For this review, take the finished solid that the model builds, in its own axes (mm). Give positions to 0.01 mm unless a question says otherwise; leave off trailing zeros. Write each loop counter-clockwise with the first axis right and the second up, starting at its lowest first coordinate (ties: lowest second). Pieces come first, ordered by that corner, then holes. Notation, with made-up numbers: (82, 72.25) -> (139, 72.25) arc R24 cw to (139, 105.25) -> close; hole circle Ø7 at (78, 54). An arc over 180 degrees is marked (long way). Answer as CSV lines item,"result".
```python
from build123d import *

# Parameters (mm, degrees)
SKETCH1_W                                          = 176.276
SKETCH1_H                                          = 49.149
BOSS_EXTRUDE1_DEPTH                                = 6.35
CUT_EXTRUDE3_DEPTH                                 = 92.719875677
CSK_FOR_10_FLAT_HEAD_MACHINE_SCREW_100_D           = 5.1054
CSK_FOR_10_FLAT_HEAD_MACHINE_SCREW_100_CSINK_D     = 9.779
CSK_FOR_10_FLAT_HEAD_MACHINE_SCREW_100_CSINK_ANGLE = 100


with BuildPart() as part:
    # Sketch1 → Boss-Extrude1 (new body)
    with BuildSketch(Plane.XY):
        Rectangle(SKETCH1_W, SKETCH1_H)
    extrude(amount=BOSS_EXTRUDE1_DEPTH)

    # Sketch22 → Cut-Extrude3 (cut, through all)
    with BuildSketch(Plane.XY.offset(6.35)):
        with BuildLine():
            ThreePointArc((-88.138, 2.504831531), (-81.209963357, 17.310760321), (-66.565807357, 24.5745))
            Line((-66.565807357, 24.5745), (-88.138, 24.5745))
            Line((-88.138, 24.5745), (-88.138, 2.504831531))
        make_face()
        with BuildLine():
            ThreePointArc((-66.565807357, -24.5745), (-81.209963357, -17.310760321), (-88.138, -2.504831531))
            Line((-88.138, -2.504831531), (-88.138, -24.5745))
            Line((-88.138, -24.5745), (-66.565807357, -24.5745))
        make_face()
        with BuildLine():
            Line((88.138, -24.5745), (88.138, -2.504831531))
            ThreePointArc((88.138, -2.504831531), (81.209963357, -17.310760321), (66.565807357, -24.5745))
            Line((66.565807357, -24.5745), (88.138, -24.5745))
        make_face()
        with BuildLine():
            Line((88.138, 24.5745), (66.565807357, 24.5745))
            ThreePointArc((66.565807357, 24.5745), (81.209963357, 17.310760321), (88.138, 2.504831531))
            Line((88.138, 2.504831531), (88.138, 24.5745))
        make_face()
    extrude(amount=-CUT_EXTRUDE3_DEPTH, mode=Mode.SUBTRACT)

    # CSK for #10 Flat Head Machine Screw (100)1 (through all)
    with Locations(Plane.XY.offset(6.35)):
        with Locations((-66.565807357, 19.4945), (-33.282903678, 19.4945), (0, 19.4945), (33.282903678, 19.4945), (66.565807357, 19.4945), (66.565807357, -19.4945), (33.282903678, -19.4945), (0, -19.4945), (-33.282903678, -19.4945), (-66.565807357, -19.4945)):
            CounterSinkHole(CSK_FOR_10_FLAT_HEAD_MACHINE_SCREW_100_D / 2, CSK_FOR_10_FLAT_HEAD_MACHINE_SCREW_100_CSINK_D / 2, counter_sink_angle=CSK_FOR_10_FLAT_HEAD_MACHINE_SCREW_100_CSINK_ANGLE)


solid = part.part
```
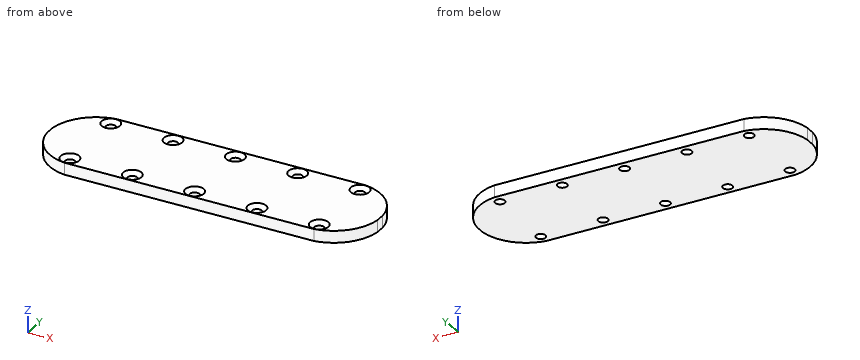
Q1. Add section A-A (x = 0). State how many separate pieces and enclosed holes the cut face has, plus the area to 3 significant figures.
Answer block:
separate pieces,"3"
enclosed holes,"0"
area,"238 mm2"
Q2. Add section C-C (y = 12). Write out the cut boundary in (x, z).
Answer block:
outline,"(-85.16, 0) -> (85.16, 0) -> (85.16, 6.35) -> (-85.16, 6.35) -> close"
Q3. To check wall thickness, follow probe 1 along Y at (x, z) = (-32, 4.5); probe 2 along X at (y, z) = (18.5, 5.25); probe 3 along Y at (x, z) = (33, 6.25). State the ranges of each line that lie inside material, in increasing order. Write a range as [from, to].
Answer block:
probe 1,"y = [-24.57, -21.85], [-17.14, 17.14], [21.85, 24.57]"
probe 2,"x = [-79.96, -70], [-63.13, -36.72], [-29.85, -3.44], [3.44, 29.85], [36.72, 63.13], [70, 79.96]"
probe 3,"y = [-24.57, -24.26], [-14.73, 14.73], [24.26, 24.57]"
Q4. Add section B-B (y = -9.5). Write out the cut boundary in (x, z), plus the area to 3 significant figures.
Answer block:
outline,"(-86.37, 0) -> (86.37, 0) -> (86.37, 6.35) -> (-86.37, 6.35) -> close"
area,"1,100 mm2"
Q5. Clearance check with flat-ended pins moving along their axes: pin 1 (1 mm diameter, centred on x = -34, y = 16, fed in from +Z); pin 2 (6 mm diameter, centred on x = 0, y = -19.49, fed in from +Z). State where each tip first meets the part, or that it passes through.
Answer block:
pin 1,"stops at z = 5.66"
pin 2,"stops at z = 4.77"
